The listing builds one solid part. Answer for the finished solid, in the listing's coordinates (mm). Face numbers are marked on the shaded views. A direction names the side the tool comes from. Round coordinates to 2 decimals unless told otherwise and drop trailing zeros. Loops run counter-clockwise (first coordinate to the right, second up) from the corner with the lowest first, then second, coordinate; pieces in that order, holes last. Notation, with made-up numbers: (73.5, 54) -> (131.5, 54) arc R27 ccw to (131.5, 87) -> close; hole circle Ø5 at (45, -15). An arc over 180 degrees is marked (long way). Write each question's results on one line, items separated by ' | '. Start each with the question number.
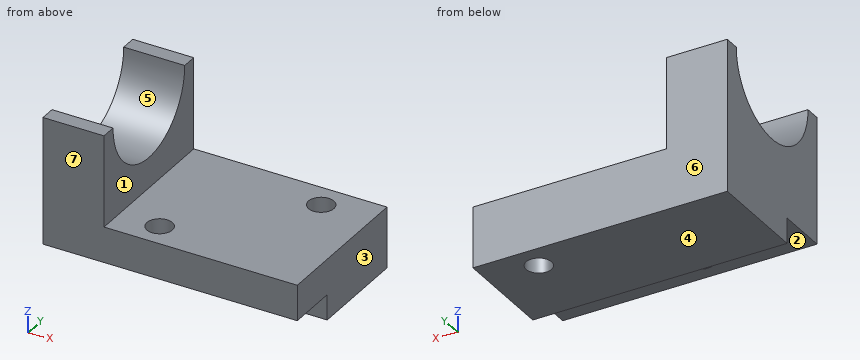
from build123d import *

# Parameters (mm, degrees)
F1_DEPTH = 100
F3_DEPTH = 24
F4_R     = 5
F5_DEPTH = 25


with BuildPart() as f1:
    # F0 (on Right) → F1 (new body)
    with BuildSketch(Plane.YZ):
        Polygon((-40, -10), (0, -10), (0, 14), (-60, 14), (-60, 0), (-40, 0), align=None)
    extrude(amount=-F1_DEPTH)

    # F2 (on face) → F3 (join)
    with BuildSketch(Plane(origin=(-100, 0, 0), x_dir=(0, -1, 0), z_dir=(-1, 0, 0))):
        with BuildLine():
            Line((0, 50), (0, 14))
            Line((0, 14), (60, 14))
            Line((60, 14), (60, 50))
            Line((60, 50), (54, 50))
            ThreePointArc((54, 50), (30, 26), (6, 50))
            Line((6, 50), (0, 50))
        make_face()
    extrude(amount=-F3_DEPTH)

    # F4 (on face) → F5 (cut)
    with BuildSketch(Plane.XY.offset(14)):
        with Locations((-20, -10)):
            Circle(F4_R)
        with Locations((-60, -50)):
            Circle(F4_R)
    extrude(amount=-F5_DEPTH, mode=Mode.SUBTRACT)


solid = f1.part
Item 1: Determine the mould class of the marked faces 4, 5, 6 and 7 for opening direction Y: +Y half, -Y half, draft (parallel to the pull), parting line (faces both ways), or undercut.
Item 2: The part is cut by section A-A, the plane x = -20. Give the vertices of the cut face in (y, z).
Item 3: Straight lines are drawn through the part: L1, parallel to Y at x = -20, z = 10; L2, parallel to Y at x = -60, z = 4; L3, parallel to X at y = -55, z = 34. For each, find the intervals that lie inside material, in ascending order. Write a range as [from, to].
Item 4: The part is cut by section B-B, the plane z = 1.5. Give the vertices of the cut face in (x, y), plus the area to 3 significant figures.
Item 5: For the marked faces 1, 2 and 3, determine the directions among +Z, -Z, +X, -X, +Y, -Y from which every point of the face is accessible in a straight line to the end or side of a thin tool.
Item 6: Each of these flat-tipped pins is pushed along its axis until it touches: pin 1 Ø11 at (y, z) = (-37, 35) entering from +X; pin 2 Ø1.5 at (x, z) = (-81, -2) entering from -Y; pin 3 Ø11.5 at (x, y) = (-60, -50) entering from -Z. Where does it stop, or does it pass through?
Item 7: The part is cut by section C-C, the plane y = -11.5. Give the vertices of the cut face in (x, z), plus the area to 3 significant figures.
Item 8: The part is cut by section D-D, the plane z = 31. Give the vertices of the cut face in (x, y).
Report:
1) face 4: draft | face 5: undercut | face 6: +Y half | face 7: -Y half
2) outline: (-60, 0) -> (-40, 0) -> (-40, -10) -> (-15, -10) -> (-15, 14) -> (-60, 14) -> close; (-5, -10) -> (0, -10) -> (0, 14) -> (-5, 14) -> close
3) L1: y = [-60, -15], [-5, 0] | L2: y = [-60, -55], [-45, 0] | L3: x = [-100, -76]
4) outline: (-100, -60) -> (0, -60) -> (0, 0) -> (-100, 0) -> close; hole circle Ø10 at (-60, -50); hole circle Ø10 at (-20, -10) | area: 5,840 mm2
5) face 1: +Z, +X, +Y, -Y | face 2: -Z, +X, -X, -Y | face 3: +Z, -Z, +X, +Y, -Y
6) pin 1: passes through | pin 2: stops at y = -40 | pin 3: stops at z = 0
7) outline: (-100, -10) -> (-24.77, -10) -> (-24.77, 14) -> (-76, 14) -> (-76, 34.71) -> (-100, 34.71) -> close; (-15.23, -10) -> (0, -10) -> (0, 14) -> (-15.23, 14) -> close | area: 2,670 mm2
8) outline: (-100, -60) -> (-76, -60) -> (-76, -44.66) -> (-100, -44.66) -> close; (-100, -15.34) -> (-76, -15.34) -> (-76, 0) -> (-100, 0) -> close
